Design review of the part built by this model. Coordinates are the model's own, in mm. A direction names the side the tool comes from. Coordinates: 2 decimals unless noted, no trailing zeros. Loops run counter-clockwise (first coordinate to the right, second up) from the corner with the lowest first, then second, coordinate; pieces in that order, holes last.
Q1. Add section C-C on z = -6. Give the boundary of the cut face in (x, y).
Q2. For P1, Ø1.7, axis at x = -3, y = -7.5, coming from the +Z side; P2, Ø4, axis at x = -5.5, z = 8.5, coming from the +Y side; P3, Ø1.5, axis at y = -1.5, z = -12.5, coming from the +X side, all flat-tipped, find the tip position at first contact; note any pin that passes through.
Q3. Machinability: for faces 1 (the face through (4.38, -8.43, -12.32)), 2 (the face through (0, 3, 15)), 3 (the face through (0, -3, 7)), which of the approach directions +Z, -Z, +X, -X, +Y, -Y give a long, thin tool a straight path to every point of the face, cutting with its end or side? Answer none if there is none.
Q4. Add section A-A on y = 0. Give the boundary of the cut face in (x, z).
Q5. Add section B-B on x = 0. Give the boundary of the cut face in (y, z), and give its area (3 significant figures).
Q6. Wall thickness on probe 1 along Z at (x, y) = (-9.5, 5.75); probe 2 along Z at (x, y) = (-0.75, -5.75); probe 3 along X at (y, z) = (-7.5, -20): over which ranges is each line inside the solid? List them lowest first.
Q7. Add section D-D on x = -7. Give the boundary of the cut face in (y, z), and give its area (3 significant figures).
```python
from build123d import *

# Parameters (mm, degrees)
F0_R     = 9.5
F1_DEPTH = 25
F2_R     = 12
F2_R_2   = 9.5
F3_DEPTH = 15
F7_DEPTH = 12.5
F8_R     = 0.8


with BuildPart() as f1:
    # F0 (on Top) → F1 (new body)
    with BuildSketch(Plane.XY):
        Circle(F0_R)
    extrude(amount=-F1_DEPTH)

    # F2 (on face) → F3 (join)
    with BuildSketch(Plane.XY):
        Circle(F2_R)
        Circle(F2_R_2, mode=Mode.SUBTRACT)
        Circle(F2_R_2)
    extrude(amount=F3_DEPTH)

    # F6 (on Right) → F7 (cut, symmetric)
    with BuildSketch(Plane.YZ):
        Polygon((-9.5, -1), (-3, -1), (-3, 15), (-12, 15), (-12, 0), (-9.5, 0), align=None)
    extrude(amount=F7_DEPTH, both=True, mode=Mode.SUBTRACT)

    # F8
    f8_edges = [f1.edges().sort_by_distance(p)[0] for p in [
        (0, -3, -1),
    ]]
    fillet(f8_edges, radius=F8_R)


solid = f1.part
```
Entries:
1. outline: circle Ø19 at (0, 0)
2. P1: stops at z = -1
2. P2: stops at y = 11.48
2. P3: stops at x = 9.47
3. face 1: -Z
3. face 2: +Z, +X, -X, +Y, -Y
3. face 3: +Z, +X, -X, -Y
4. outline: (-12, 0) - (-9.5, 0) - (-9.5, -25) - (9.5, -25) - (9.5, 0) - (12, 0) - (12, 15) - (-12, 15) - close
5. outline: (-9.5, -25) - (9.5, -25) - (9.5, 0) - (12, 0) - (12, 15) - (-3, 15) - (-3, -0.2) arc R0.8 cw to (-3.8, -1) - (-9.5, -1) - close
5. area: 694 mm2
6. probe 1: z = 0 to 15
6. probe 2: z = -25 to -1
6. probe 3: x = -5.83 to 5.83
7. outline: (-6.42, -25) - (6.42, -25) - (6.42, 0) - (9.75, 0) - (9.75, 15) - (-3, 15) - (-3, -0.2) arc R0.8 cw to (-3.8, -1) - (-6.42, -1) - close
7. area: 509 mm2
